Geometry check sheet. Reference: the model listing, model coordinates, mm. Round coordinates to 2 decimals unless told otherwise and drop trailing zeros. Order: outer loops, then holes, each group sorted by start corner. A loop starts at its lowest first (then second) coordinate and runs counter-clockwise, first axis right, second up. Notation, with made-up numbers: (59, 14) - (88, 14) arc R22 ccw to (88, 43) - close; hole circle Ø6 at (16.25, -31). An arc over 180 degrees is marked (long way). Return JSON: item names as keys, results as strings. Group by question number.
Q1. Sectioned sample at C-C, the plane z = -38. Record the cut outline in (x, y).
Q2. Sectioned sample at B-B, the plane x = 0.45. Give the number of separate pieces and of enclosed holes in the cut face, then the cut area to 3 significant figures.
Q3. Material ranges on line 1 along Z through (x, y) = (0.7, -5.08); line 2 along Z through (x, y) = (0.65, 1); line 3 along Z through (x, y) = (0.6, 20.5), recorded low to high.
Q4. Sectioned sample at A-A, the plane y = 18.5. Record the cut outline in (x, z).
Q5. Draft check along Y on faces 1 (the cylindrical face through (0.78, -0.11, 4.85)), 2 (the cylindrical face through (0.8, 36.1, -31.2)), 3 (the flat face through (0, 10, -43)). Enter one of: pulls with the +Y half, pulls with the -Y half, needs draft (parallel to the pull), parting line crosses it, or undercut.
Q6. Sectioned sample at D-D, the plane y = 25.5. Record the cut outline in (x, z).
Q7. Gauge pin test, flat ends, axial feed: pin 1 Ø4 at (y, z) = (19.46, -42.55) entering from +X; pin 2 Ø6 at (y, z) = (36.74, -41.6) entering from +X. Record the tip position at first contact, or that the pin passes through.
Autodesk Inventor part; units mm, degrees
ref_plane "YZ Plane" through (0, 0, 0) normal (1, 0, 0) x (0, 1, 0)
ref_plane "XZ Plane" through (0, 0, 0) normal (0, 1, 0) x (-1, 0, 0)
ref_plane "XY Plane" through (0, 0, 0) normal (0, 0, 1) x (1, 0, 0)
sketch "Sketch4" plane through (0, 0, 0) normal (1, 0, 0) x (0, 1, 0)
  line L0 (-0.177, -66.4213) -> (-12.877, -66.4213)
  line L1 (0, -49.1236) -> (-5.08, -49.1236)
  circle A0 centre (-5.08, -49.1236) radius 2.1209
  line L2 (-5.08, -49.1236) -> (7.1876, -45.838)
  arc A1 (-12.7, -31.6611) -> (-12.877, -66.4213) centre (3.3882, -49.1236) ccw
  circle A2 centre (7.1876, -45.838) radius 2.3114
  arc A3 (-12.877, -66.4213) -> (38.1002, -29.2262) centre (9.1157, -43.0325) ccw
  circle A4 centre (19.4552, -42.5523) radius 2.3114
  line L3 (7.1876, -45.838) -> (19.4552, -42.5523)
  line L4 (38.1695, -29.2174) -> (33.9062, -30.4753)
  circle A5 centre (34.972, -52.8945) radius 2.3114
  circle A6 centre (36.7356, -41.6045) radius 2.3114
  arc A7 (39.2694, -49.6585) -> (39.5231, -48.5235) centre (33.2252, -47.7117) ccw
  line L5 (39.2474, -54.1108) -> (34.972, -52.8945)
  line L6 (41.1789, -41.481) -> (36.7356, -41.6045)
  circle A8 centre (33.9062, -30.4753) radius 2.3114
  arc A9 (38.1002, -29.2262) -> (32.6481, -26.212) centre (33.2894, -31.4901) ccw
  line L7 (33.9062, -30.4753) -> (32.6481, -26.212)
  arc A10 (-12.7, -31.6611) -> (-4.8514, 0) centre (-31.4487, -10.21) ccw
  line L8 (2.3114, 0) -> (4.8514, 0)
  arc A11 (4.8514, 0) -> (0, 4.8514) centre (0, 0) ccw
  arc A12 (0, 4.8514) -> (-4.8514, 0) centre (0, 0) ccw
  arc A13 (4.8514, 0) -> (32.6481, -26.212) centre (41.1134, 10.6096) ccw
  circle A14 centre (0, 0) radius 2.1209
  circle A15 centre (2.1209, -9.1751) radius 2.3114
  point P0 (38.105, -29.2364)
  point P1 (36.1231, -29.8211)
  point P2 (33.2519, -28.2584)
  dimension "d110" = 2.54
  dimension "d111" = 4.8514
  dimension "d112" = 5.08
  dimension "d113" = 12.7
  dimension "d114" = 6.35
  dimension "d115" = 4.445
  dimension "d116" = 4.6228
  dimension "d117" = 4.2418
  dimension "d118" = 4.445
  dimension "d119" = 12.7
  dimension "d120" = 12.7
  dimension "d121" = 4.6228
  dimension "d122" = 4.6228
  dimension "d123" = 4.445
  dimension "d124" = 4.6228
  dimension "d125" = 4.445
  dimension "d126" = 4.6228
  dimension "d127" = 4.2418
  dimension "d128" = 4.6228
extrude "Extrusion4" add sketch "Sketch4" along normal blind 1.5875 contours A10 A12 A11 A13 L7 A8 L4 A3 A1 | L4 A8 L7 A9 A3
properties part number "Odom Pod Poly" material "Polycarbonate, Clear"
Reply:
{
 "1": {"outline": "(0, -17.59) - (1.59, -17.59) - (1.59, 40.82) - (0, 40.82) - close"},
 "2": {"separate pieces": "1", "enclosed holes": "8", "area": "2,880 mm^2"},
 "3": {"line 1": "-71.83 to -51.24, -47 to -21", "line 2": "-74.09 to -11.2, -7.15 to -1.87, 1.87 to 4.75", "line 3": "-73.05 to -44.61, -40.49 to -21.05"},
 "4": {"outline": "(0, -73.74) - (1.59, -73.74) - (1.59, -44.66) - (0, -44.66) - close; (0, -40.45) - (1.59, -40.45) - (1.59, -19.66) - (0, -19.66) - close"},
 "5": {"face 1": "parting line crosses it", "face 2": "undercut", "face 3": "needs draft"},
 "6": {"outline": "(0, -70.64) - (1.59, -70.64) - (1.59, -23.8) - (0, -23.8) - close"},
 "7": {"pin 1": "through", "pin 2": "x = 1.59"}
}
